The figure shows three views and two pictorial views of one solid part (mm, origin at its lowest corner). Answer the questions. Round coordinates to 2 decimals unless told otherwise and drop trailing zeros. Loops run counter-clockwise (first coordinate to the right, second up) from the corner with the lowest first, then second, coordinate; pieces in that order, holes last. Notation, with made-up numbers: (84, 17) - (101, 17) arc R10 cw to (101, 21) - close; hole circle Ø11 at (-19, 10). An arc over 180 degrees is marked (long way). Use one line per item in the form item = value. Start each with the question number.
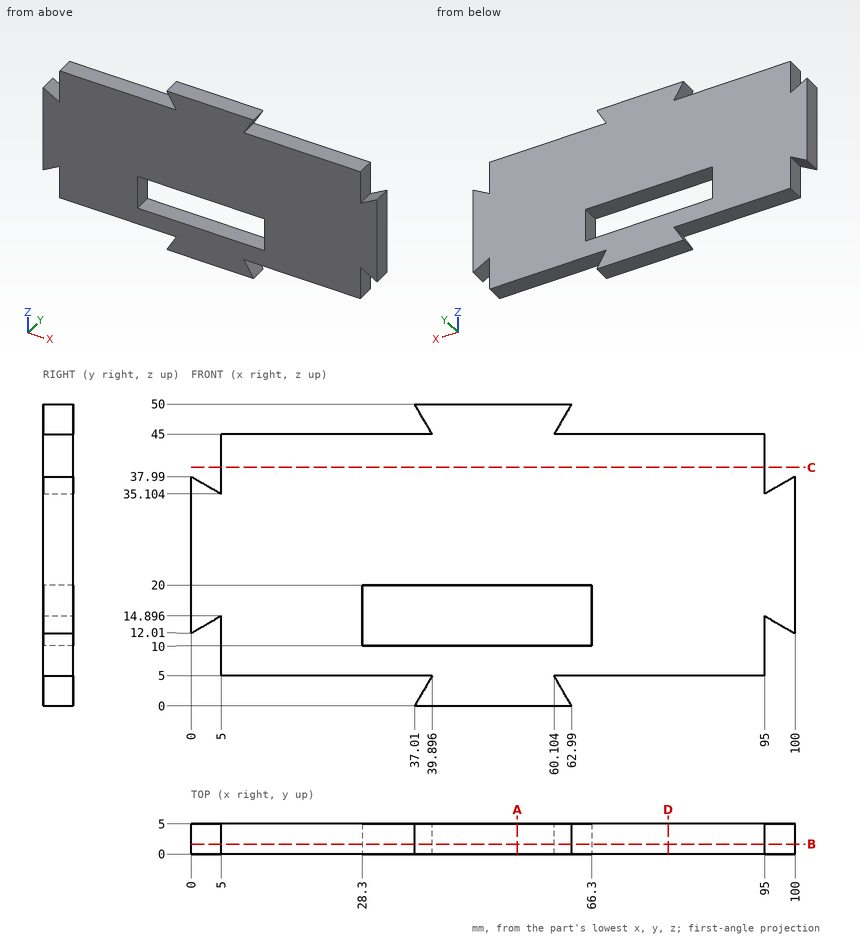
1) A cutting plane is placed at B-B on y = 1.65. Write down the section's boundary in (x, z), plus the area to 3 significant figures.
2) A cutting plane is placed at D-D on x = 79. Write down the section's boundary in (y, z), plus the area to 3 significant figures.
3) A cutting plane is placed at C-C on z = 39.5. Write down the section's boundary in (x, y).
4) Flat-ended cylindrical pins translate along their axes: pin 1 (1.5 mm diameter, centred on y = 1.5, z = 11, fed in from +X); pin 2 (2.5 mm diameter, centred on x = 71.5, y = 2.5, fed in from -Z); pin 3 (2.5 mm diameter, centred on x = 25.5, y = 1.5, fed in from +Z). Find the tip coordinate at first contact, or state that the pin passes through.
5) Straight lines are drawn through the part: line 1 (X direction, y = 2.15, z = 16); line 2 (Z direction, x = 34.5, y = 2.2); line 3 (Z direction, x = 38, y = 1.1) (1 decimal). For each, find the intervals that lie inside material, in ascending order. Write a range as from..to.
6) A cutting plane is placed at A-A on x = 54. Write down the section's boundary in (y, z), plus the area to 3 significant figures.
Checks:
q1.outline = (0, 12.01) - (5, 14.9) - (5, 5) - (39.9, 5) - (37.01, 0) - (62.99, 0) - (60.1, 5) - (95, 5) - (95, 14.9) - (100, 12.01) - (100, 37.99) - (95, 35.1) - (95, 45) - (60.1, 45) - (62.99, 50) - (37.01, 50) - (39.9, 45) - (5, 45) - (5, 35.1) - (0, 37.99) - close; hole (28.3, 10) - (66.3, 10) - (66.3, 20) - (28.3, 20) - close
q1.area = 3,680 mm²
q2.outline = (0, 5) - (5, 5) - (5, 45) - (0, 45) - close
q2.area = 200 mm²
q3.outline = (5, 0) - (95, 0) - (95, 5) - (5, 5) - close
q4.pin_1 = 95
q4.pin_2 = 5
q4.pin_3 = 45
q5.line_1 = 0..28.3, 66.3..100
q5.line_2 = 5..10, 20..45
q5.line_3 = 0..1.7, 5..10, 20..45, 48.3..50
q6.outline = (0, 0) - (5, 0) - (5, 10) - (0, 10) - close; (0, 20) - (5, 20) - (5, 50) - (0, 50) - close
q6.area = 200 mm²
